```python
from build123d import *

# Parameters (mm, degrees)
SKETCH_1_R             = 19
SKETCH_1_R_2           = 7.5
EXTRUDE_1_DEPTH        = 32
SKETCH_2_R             = 9.5
CUT_EXTRUDE_1_DEPTH    = 5
CUT_EXTRUDE_START      = -5
SKETCH_3_R             = 9.5
CUT_EXTRUDE_2_DEPTH    = 5
HOLE_WIZARD_M4_1_D     = 3.3
HOLE_WIZARD_M4_1_DEPTH = 10.1
HOLE_WIZARD_M4_1_TIP   = 0.991420021
HOLE_WIZARD_M4_2_D     = 3.3
HOLE_WIZARD_M4_2_DEPTH = 10.1
HOLE_WIZARD_M4_2_TIP   = 0.991420021


with BuildPart() as part:
    # 草图1 → 凸台-拉伸1 (new body)
    with BuildSketch(Plane(origin=(0, 0, 0), x_dir=(1, 0, 0), z_dir=(0, 1, 0))):
        with Locations(Location((0, 0, 0), (0, 0, 270))):
            Circle(SKETCH_1_R)
        with Locations(Location((0, 0, 0), (0, 0, 270))):
            Circle(SKETCH_1_R_2, mode=Mode.SUBTRACT)
    extrude(amount=EXTRUDE_1_DEPTH)

    # 草图2 → 切除-拉伸1 (cut)
    with BuildSketch(Plane(origin=(0, 32, 0), x_dir=(1, 0, 0), z_dir=(0, 1, 0))):
        with Locations(Location((0, 0, 0), (0, 0, 270))):
            Circle(SKETCH_2_R)
    extrude(amount=-CUT_EXTRUDE_1_DEPTH, mode=Mode.SUBTRACT)

    # 草图3 → 切除-拉伸2 (cut)
    with BuildSketch(Plane.XZ.offset(CUT_EXTRUDE_START)):
        with Locations(Location((0, 0, 0), (0, 0, 90))):
            Circle(SKETCH_3_R)
    extrude(amount=CUT_EXTRUDE_2_DEPTH, mode=Mode.SUBTRACT)

    # M4 螺纹孔1
    with Locations(Plane.XZ):
        with Locations((0, -14), (-14, 0), (0, 14), (14, 0)):
            Hole(HOLE_WIZARD_M4_1_D / 2, depth=HOLE_WIZARD_M4_1_DEPTH)
            with Locations((0, 0, -(HOLE_WIZARD_M4_1_DEPTH + HOLE_WIZARD_M4_1_TIP / 2))):  # 118° drill point
                Cone(0, HOLE_WIZARD_M4_1_D / 2, HOLE_WIZARD_M4_1_TIP, mode=Mode.SUBTRACT)

    # M4 螺纹孔2
    with Locations(Plane(origin=(0, 32, 0), x_dir=(-1, 0, 0), z_dir=(0, 1, 0))):
        with Locations((-14, 0), (0, 14), (14, 0), (0, -14)):
            Hole(HOLE_WIZARD_M4_2_D / 2, depth=HOLE_WIZARD_M4_2_DEPTH)
            with Locations((0, 0, -(HOLE_WIZARD_M4_2_DEPTH + HOLE_WIZARD_M4_2_TIP / 2))):  # 118° drill point
                Cone(0, HOLE_WIZARD_M4_2_D / 2, HOLE_WIZARD_M4_2_TIP, mode=Mode.SUBTRACT)


solid = part.part
```
The model under review builds one solid part; all positions refer to its coordinate system, in mm. A direction names the side the tool comes from. Give positions to 0.01 mm unless a question says otherwise; leave off trailing zeros. Write each loop counter-clockwise with the first axis right and the second up, starting at its lowest first coordinate (ties: lowest second). Pieces come first, ordered by that corner, then holes. Notation, with made-up numbers: (-22.5, 88) -> (3.5, 88) arc R29 ccw to (3.5, 113) -> close; hole circle Ø7 at (54, -36). An arc over 180 degrees is marked (long way). Answer in a Markdown table with one row per item.
1) Add section C-C on y = 15.5. State the section outline as (x, z) points.
Worked answers:
| item | result |
|---|---|
| outline | circle Ø38 at (0, 0); hole circle Ø15 at (0, 0) |
2) Mouldability with a two-part tool opening along Z and no side actions: class faces 4 (the flat face through (-4, 32, -9)), 5 (the cylindrical face through (-11.56, 15.78, -15.08)), 6 (the flat face through (-8, 5, 1)) as +Z half, -Z half, draft (parallel to the pull), parting line (faces both ways), or undercut.
Worked answers:
| item | result |
|---|---|
| face 4 | draft |
| face 5 | parting line |
| face 6 | undercut |
3) Add section B-B on z = 5. State the section outline as (x, y) points, plus the area to 3 significant figures.
Worked answers:
| item | result |
|---|---|
| outline | (-18.33, 0) -> (-8.08, 0) -> (-8.08, 5) -> (-5.59, 5) -> (-5.59, 27) -> (-8.08, 27) -> (-8.08, 32) -> (-18.33, 32) -> close; (5.59, 5) -> (8.08, 5) -> (8.08, 0) -> (18.33, 0) -> (18.33, 32) -> (8.08, 32) -> (8.08, 27) -> (5.59, 27) -> close |
| area | 766 mm² |
4) For L1, parallel to X at y = 3.2, z = 0; L2, parallel to X at y = 24.5, z = 0; L3, parallel to Z at x = -1, y = 3, list the stretches that pass through material, from the lowest coordinate up. Write a range as [from, to].
Worked answers:
| item | result |
|---|---|
| L1 | [-19, -15.65], [-12.35, -9.5], [9.5, 12.35], [15.65, 19] |
| L2 | [-19, -15.65], [-12.35, -7.5], [7.5, 12.35], [15.65, 19] |
| L3 | [-18.97, -15.31], [-12.69, -9.45], [9.45, 12.69], [15.31, 18.97] |
5) Add section D-D on z = -5.5. State the section outline as (x, y) points.
Worked answers:
| item | result |
|---|---|
| outline | (-18.19, 0) -> (-7.75, 0) -> (-7.75, 5) -> (-5.1, 5) -> (-5.1, 27) -> (-7.75, 27) -> (-7.75, 32) -> (-18.19, 32) -> close; (5.1, 5) -> (7.75, 5) -> (7.75, 0) -> (18.19, 0) -> (18.19, 32) -> (7.75, 32) -> (7.75, 27) -> (5.1, 27) -> close |
6) Clearance check with flat-ended pins moving along their axes: P1, Ø1.5, axis at y = 22, z = 12.5, coming from the -X side; P2, Ø8, axis at x = 11.5, y = 4, coming from the -Z side; P3, Ø2, axis at y = 3.5, z = -5.5, coming from the -X side. State where each tip first meets the part, or that it passes through.
Worked answers:
| item | result |
|---|---|
| P1 | x = -14.93 |
| P2 | z = -17.46 |
| P3 | x = -18.46 |
7) Tool access review of faces 1 (the cylindrical face through (0.215, 5.121, -12.364)), 2 (the cylindrical face through (0.33, 15.846, -7.493)), 3 (the cylindrical face through (-1.216, 26.879, 15.115)): name each direction out of +Z, -Z, +X, -X, +Y, -Y from which nothing blocks a thin tool from reaching the whole face with its end or side.
Worked answers:
| item | result |
|---|---|
| face 1 | -Y |
| face 2 | +Y, -Y |
| face 3 | +Y |
8) Add section A-A on y = 6.5. State the section outline as (x, z) points, plus the area to 3 significant figures.
Worked answers:
| item | result |
|---|---|
| outline | circle Ø38 at (0, 0); hole circle Ø3.3 at (-14, 0); hole circle Ø15 at (0, 0); hole circle Ø3.3 at (0, -14); hole circle Ø3.3 at (0, 14); hole circle Ø3.3 at (14, 0) |
| area | 923 mm² |
